```python
from build123d import *

# Parameters (mm, degrees)
EXTRUDE_1_DEPTH     = 15
SKETCH_5_R          = 15
EXTRUDE_2_DEPTH     = 17
SKETCH_7_R          = 10
CUT_EXTRUDE_1_DEPTH = 2


with BuildPart() as part:
    # ｽｹｯﾁ4 → ﾎﾞｽ - 押し出し1 (new body)
    with BuildSketch(Plane.XY):
        with BuildLine():
            Line((-53.623111018, -124.995132678), (-58.940636287, -129.45706617))
            ThreePointArc((-58.940636287, -129.45706617), (-60.005384698, -131.552012131), (-59.233530865, -133.771635843))
            ThreePointArc((-59.233530865, -133.771635843), (57.362306223, -135.763481103), (52.076178918, -19.270504783))
            Line((52.076178918, -19.270504783), (10.606601718, 10.606601718))
            ThreePointArc((10.606601718, 10.606601718), (-10.606601718, 10.606601718), (-10.606601718, -10.606601718))
            Line((-10.606601718, -10.606601718), (14.536280154, -62.889638219))
            ThreePointArc((14.536280154, -62.889638219), (14.918089499, -66.109676181), (13.244185189, -68.886809092))
            Line((13.244185189, -68.886809092), (-53.623111018, -124.995132678))
        make_face()
        with BuildLine():
            Line((21.232400696, -76.813798404), (45.844843506, -127.993820346))
            ThreePointArc((45.844843506, -127.993820346), (46.221944165, -131.235480845), (44.518718993, -134.019289696))
            ThreePointArc((44.518718993, -134.019289696), (-2.231208213, -149.964431749), (-47.870174388, -131.072951785))
            ThreePointArc((-47.870174388, -131.072951785), (-48.817477846, -128.802229421), (-47.747678417, -126.586582094))
            Line((-47.747678417, -126.586582094), (13.511229465, -75.151532228))
            ThreePointArc((13.511229465, -75.151532228), (17.77869109, -74.092739753), (21.232400696, -76.813798404))
        make_face(mode=Mode.SUBTRACT)
    extrude(amount=EXTRUDE_1_DEPTH)

    # ｽｹｯﾁ5 → ﾎﾞｽ - 押し出し2 (add)
    with BuildSketch(Plane.XY.offset(15)):
        with Locations(Location((0, 0, 0), (0, 0, 225))):
            Circle(SKETCH_5_R)
    extrude(amount=EXTRUDE_2_DEPTH)

    # ｽｹｯﾁ7 → ｶｯﾄ - 押し出し1 (cut)
    with BuildSketch(Plane.XY.offset(32)):
        Circle(SKETCH_7_R)
    extrude(amount=-CUT_EXTRUDE_1_DEPTH, mode=Mode.SUBTRACT)


solid = part.part
```
Geometry: final body of the model. Coordinates: model frame, mm. A direction names the side the tool comes from. Coordinates: 2 decimals unless noted, no trailing zeros. Order: outer loops, then holes, each group sorted by start corner. A loop starts at its lowest first (then second) coordinate and runs counter-clockwise, first axis right, second up. Notation, with made-up numbers: (75, -10) - (104, -10) arc R25 cw to (104, 18) - close; hole circle Ø2 at (86, -11). An arc over 180 degrees is marked (long way). Write each question's results on one line, items separated by ' | '.
1) Section A-A, the plane z = 9. Return loops of the section in (x, y), plus the area to 3 significant figures.
Results list:
outline: (-59.23, -133.77) arc R80 ccw (long way) to (52.08, -19.27) - (10.61, 10.61) arc R15 ccw to (-10.61, -10.61) - (14.54, -62.89) arc R5 cw to (13.24, -68.89) - (-58.94, -129.46) arc R3 ccw to start; hole (-47.87, -131.07) arc R70 ccw to (44.52, -134.02) arc R5 ccw to (45.84, -127.99) - (21.23, -76.81) arc R5 ccw to (13.51, -75.15) - (-47.75, -126.59) arc R3 ccw to start | area: 8,940 mm^2
2) Line query: line 1 (Y direction, x = 0, z = 31.05); line 2 (Z direction, x = 48, y = -74); line 3 (Z direction, x = -1, y = 5.5). Output: solid intervals per line, ascending. Write a range as from..to.
Results list:
line 1: -15..-10, 10..15 | line 2: 0..15 | line 3: 0..30
3) Section C-C, the plane y = -97.5. Return loops of the section in (x, z).
Results list:
outline: (-20.86, 0) - (-13.11, 0) - (-13.11, 15) - (-20.86, 15) - close; (31.18, 0) - (78.06, 0) - (78.06, 15) - (31.18, 15) - close
4) Set-up query: faces 1 (the flat face through (-9, -5, 32)), 2 (the flat face through (1.79, -36.38, 7.4)), 3 (the cylindrical face through (-48.82, -128.84, 7.4)), 4 (the cylindrical face through (-8.06, 12.65, 19.33)), 5 (the flat face through (25, -71, 0)). Return all of +Z, -Z, +X, -X, +Y, -Y with unobstructed straight access to the full face (end or side cutting, diameter ignored); none if empty.
Results list:
face 1: +Z, +X, -X, +Y, -Y | face 2: +Z, -Z, -X | face 3: +Z, -Z | face 4: +Z | face 5: -Z, +X, -X, +Y, -Y
5) Pin query (flat end, axial travel): pin 1 (16 mm diameter, centred on x = 0, y = 0, fed in from +Z); pin 2 (5 mm diameter, centred on x = -5.5, z = 18, fed in from -Y); pin 3 (8 mm diameter, centred on y = -79, z = 7.5, fed in from -X). Return the tip coordinate at first contact, or that it passes through.
Results list:
pin 1: z = 30 | pin 2: y = -14.7 | pin 3: x = -3.58
6) Section B-B, the plane x = 0. Return loops of the section in (y, z), plus the area to 3 significant figures.
Results list:
outline: (-160, 0) - (-150, 0) - (-150, 15) - (-160, 15) - close; (-86.5, 0) - (-80, 0) - (-80, 15) - (-86.5, 15) - close; (-32.66, 0) - (15, 0) - (15, 32) - (10, 32) - (10, 30) - (-10, 30) - (-10, 32) - (-15, 32) - (-15, 15) - (-32.66, 15) - close | area: 1,430 mm^2
7) Section D-D, the plane x = 39.5. Return loops of the section in (y, z).
Results list:
outline: (-149.57, 0) - (-137.79, 0) - (-137.79, 15) - (-149.57, 15) - close; (-114.8, 0) - (-10.21, 0) - (-10.21, 15) - (-114.8, 15) - close
